Verification items for this drawing (mm, ordinates from the low corner). A direction names the side the tool comes from. Round coordinates to 2 decimals unless told otherwise and drop trailing zeros. Loops run counter-clockwise (first coordinate to the right, second up) from the corner with the lowest first, then second, coordinate; pieces in that order, holes last. Notation, with made-up numbers: (58.25, 37) -> (90.25, 37) arc R29 cw to (90.25, 67) -> close; hole circle Ø8 at (-34.5, 63.25). An arc over 180 degrees is marked (long way). One line per item, written item: value. Start each with the question number.
1. Release check for a two-part mould opening along Z. For the marked faces 3, 4 and 5 record: +Z half, -Z half, draft (parallel to the pull), parting line (faces both ways), or undercut.
2. Cross-section at B-B on z = 62.5. Record the cut outline in (x, y), then the cut area to 3 significant figures.
3. Cross-section at A-A on y = 1.5. Record the cut outline in (x, z).
4. Cross-section at C-C on x = 21. Record the cut outline in (y, z).
5. Go/stop test with a flat-tipped pin: pin 1 (17.5 mm diameter, centred on x = 29, z = 41.5, fed in from -Y). Record where the tip stops, or that it passes through.
6. Material ranges on L1, parallel to X at y = 2, z = 30.5; L2, parallel to Z at x = 37, y = 5.75; L3, parallel to Y at x = 16, z = 30.5, recorded low to high.
7. Set-up check for the marked faces 1 and 2: record each of +Z, -Z, +X, -X, +Y, -Y from which the full face is reachable in a straight line by a thin tool's end or side.
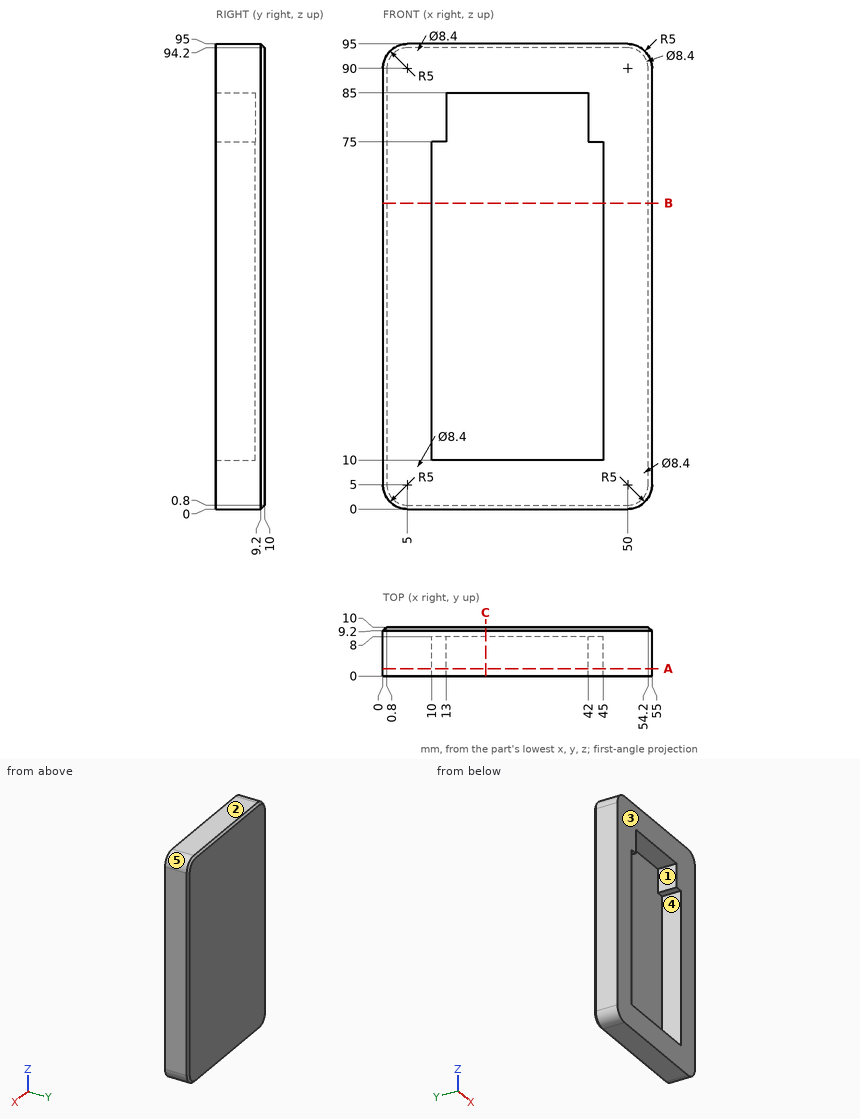
Taken from the geometry:
1. face 3: draft
1. face 4: undercut
1. face 5: +Z half
2. outline: (0, 0) -> (10, 0) -> (10, 8) -> (45, 8) -> (45, 0) -> (55, 0) -> (55, 9.2) -> (54.2, 10) -> (0.8, 10) -> (0, 9.2) -> close
2. area: 269 mm2
3. outline: (0, 5) arc R5 ccw to (5, 0) -> (50, 0) arc R5 ccw to (55, 5) -> (55, 90) arc R5 ccw to (50, 95) -> (5, 95) arc R5 ccw to (0, 90) -> close; hole (10, 10) -> (45, 10) -> (45, 75) -> (42, 75) -> (42, 85) -> (13, 85) -> (13, 75) -> (10, 75) -> close
4. outline: (0, 0) -> (9.2, 0) -> (10, 0.8) -> (10, 94.2) -> (9.2, 95) -> (0, 95) -> (0, 85) -> (8, 85) -> (8, 10) -> (0, 10) -> close
5. pin 1: stops at y = 8
6. L1: x = 0 to 10, 45 to 55
6. L2: z = 0 to 10, 85 to 95
6. L3: y = 8 to 10
7. face 1: -Y
7. face 2: +Z, +X, -X, +Y, -Y
